Part print with two shaded views. Sizes in mm from the minimum x, y, z corner. Round coordinates to 2 decimals unless told otherwise and drop trailing zeros. Order: outer loops, then holes, each group sorted by start corner. A loop starts at its lowest first (then second) coordinate and runs counter-clockwise, first axis right, second up. Notation, with made-up numbers: M 55,9 L 92,9 A28 ccw 92,27 Z; hole C 63.5,88.25 d7. An arc over 180 degrees is marked long. Return JSON: item names as keys, results as strings. Group by question number.
Item 1: Probe line 1 along Z through (x, y) = (10, 22.25); line 2 along Z through (x, y) = (11.75, 22.25); line 3 along X through (y, z) = (11, 30). List the from-to ranges inside material, lowest first.
Item 2: Slice it at A-A on z = 10. Write the cut outline in (x, y).
Item 3: Pin check, flat tip, straight feed: pin 1 Ø4 at (x, z) = (4.5, 35.5) entering from -Y. Stop position of the tip, or through.
Item 4: Slice it at D-D on y = 3.75. Write the cut outline in (x, z).
Item 5: Slice it at B-B on y = 23. Write the cut outline in (x, z).
Item 6: Pull direction X, two halves, no side cores. Call the marked faces 1, 2, 3 and 4: pulls with the +X half, pulls with the -X half, needs draft (parallel to the pull), parting line crosses it, or undercut.
Item 7: Slice it at C-C on z = 14.5. Write the cut outline in (x, y).
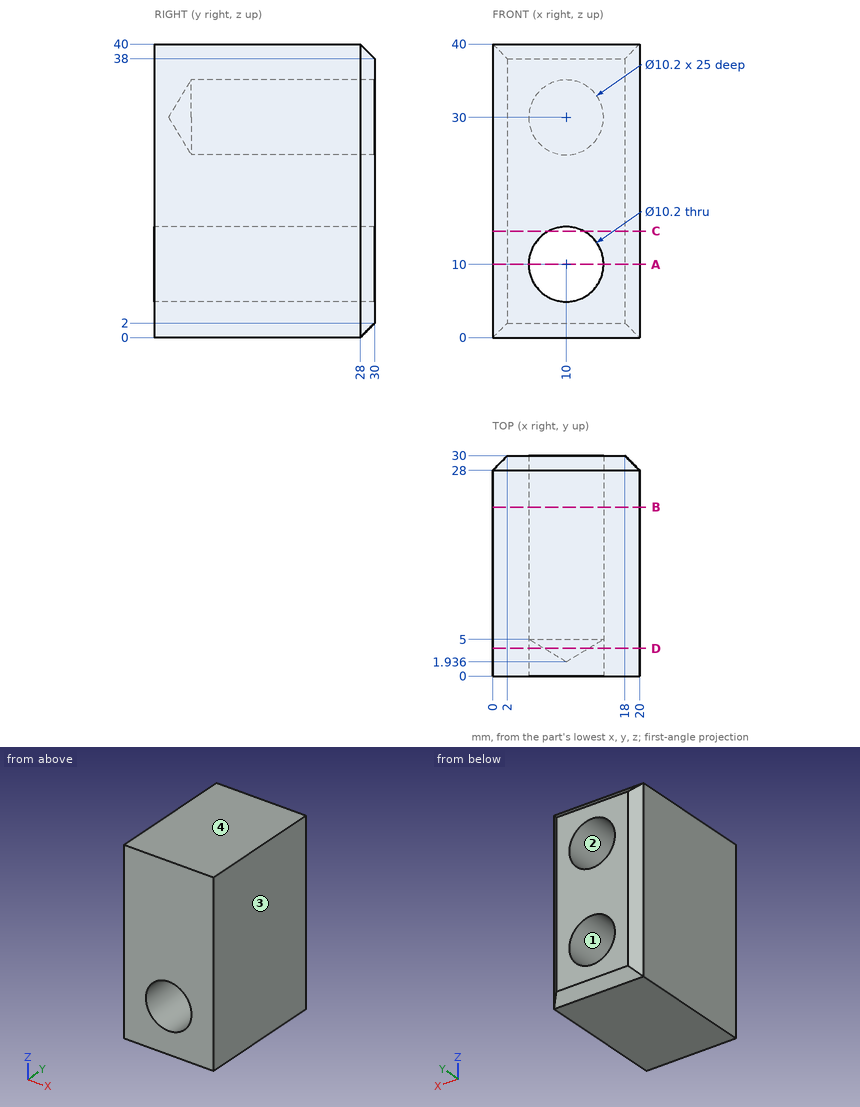
Output values:
{
 "1": {"line 1": "0 to 4.9, 15.1 to 24.9, 35.1 to 40", "line 2": "0 to 5.21, 14.79 to 25.21, 34.79 to 40", "line 3": "0 to 4.9, 15.1 to 20"},
 "2": {"outline": "M 0,0 L 4.9,0 L 4.9,30 L 2,30 L 0,28 Z; M 15.1,0 L 20,0 L 20,28 L 18,30 L 15.1,30 Z"},
 "3": {"pin 1": "y = 0"},
 "4": {"outline": "M 0,0 L 20,0 L 20,40 L 0,40 Z; hole C 10,10 d10.2; hole C 10,30 d6.04"},
 "5": {"outline": "M 0,0 L 20,0 L 20,40 L 0,40 Z; hole C 10,10 d10.2; hole C 10,30 d10.2"},
 "6": {"face 1": "undercut", "face 2": "undercut", "face 3": "pulls with the +X half", "face 4": "needs draft"},
 "7": {"outline": "M 0,0 L 7.6,0 L 7.6,30 L 2,30 L 0,28 Z; M 12.4,0 L 20,0 L 20,28 L 18,30 L 12.4,30 Z"}
}
